```python
from build123d import *

# Parameters (mm, degrees)
SKETCH1_W          = 66.04
SKETCH1_H          = 102.87
EXTRUDE1_DEPTH     = 25.2476
FILLET1_R          = 2.54
SKETCH2_R          = 0.3175
EXTRUDE2_DEPTH     = 5.334
LPATTERN1_COUNT    = 25
LPATTERN1_PITCH    = 2.54
SKETCH3_R          = 0.3175
EXTRUDE3_DEPTH     = 5.334
LPATTERN2_COUNT    = 16
LPATTERN2_PITCH    = 2.54
CUT_EXTRUDE1_START = -5.334
CUT_EXTRUDE1_DEPTH = 5.334
SKETCH5_R          = 2.7051
CUT_EXTRUDE2_DEPTH = 25.654


with BuildPart() as part:
    # Sketch1 → Extrude1 (new body)
    with BuildSketch(Plane(origin=(0, 0, 0), x_dir=(1, 0, 0), z_dir=(0, 1, 0))):
        with Locations((33.02, 51.435)):
            Rectangle(SKETCH1_W, SKETCH1_H)
    extrude(amount=EXTRUDE1_DEPTH)

    # Fillet1
    fillet1_edges = [part.edges().sort_by_distance(p)[0] for p in [
        (0, 12.6238, -102.87),
        (66.04, 12.6238, -102.87),
        (66.04, 12.6238, 0),
        (0, 12.6238, 0),
    ]]
    fillet(fillet1_edges, radius=FILLET1_R)

    # Sketch2 → Extrude2 (add)
    with BuildSketch(Plane.XZ):
        with Locations(Location((56.1848, -20.955, 0), (0, 0, 270))):
            Circle(SKETCH2_R)
        with Locations(Location((58.7248, -20.955, 0), (0, 0, 270))):
            Circle(SKETCH2_R)
    extrude2 = extrude(amount=EXTRUDE2_DEPTH)

    # LPattern1: Extrude2 ×25
    with Locations(*[(0, 0, -i * LPATTERN1_PITCH) for i in range(1, LPATTERN1_COUNT)]):
        add(extrude2)

    # Sketch3 → Extrude3 (add)
    with BuildSketch(Plane.XZ):
        with Locations(Location((8.4328, -69.215, 0), (0, 0, 270))):
            Circle(SKETCH3_R)
        with Locations(Location((10.9728, -69.215, 0), (0, 0, 270))):
            Circle(SKETCH3_R)
    extrude3 = extrude(amount=EXTRUDE3_DEPTH)

    # LPattern2: Extrude3 ×16
    with Locations(*[(0, 0, i * LPATTERN2_PITCH) for i in range(1, LPATTERN2_COUNT)]):
        add(extrude3)

    # Sketch4 → Cut-Extrude1 (cut)
    with BuildSketch(Plane.XZ.offset(CUT_EXTRUDE1_START)):
        with BuildLine():
            Line((53.34, 0), (63.5, 0))
            ThreePointArc((63.5, 0), (65.296051224, -0.743948776), (66.04, -2.54))
            Line((66.04, -2.54), (66.04, -12.7))
            ThreePointArc((66.04, -12.7), (56.838081011, -9.201918989), (53.34, 0))
        make_face()
        with BuildLine():
            Line((12.7, -102.87), (2.54, -102.87))
            ThreePointArc((2.54, -102.87), (0.743948776, -102.126051224), (0, -100.33))
            Line((0, -100.33), (0, -90.17))
            ThreePointArc((0, -90.17), (9.206362116, -93.663637884), (12.7, -102.87))
        make_face()
    extrude(amount=CUT_EXTRUDE1_DEPTH, mode=Mode.SUBTRACT)

    # Sketch5 → Cut-Extrude2 (cut)
    with BuildSketch(Plane.XZ):
        with Locations(Location((33.5788, -5.969, 0), (0, 0, 270))):
            Circle(SKETCH5_R)
        with Locations(Location((33.5788, -94.361, 0), (0, 0, 270))):
            Circle(SKETCH5_R)
    extrude(amount=-CUT_EXTRUDE2_DEPTH, mode=Mode.SUBTRACT)


solid = part.part
```
Check sheet for the modelled part. Datum: model origin and axes. Units: mm. A direction names the side the tool comes from. Coordinates: 2 decimals unless noted, no trailing zeros. Order: outer loops, then holes, each group sorted by start corner. A loop starts at its lowest first (then second) coordinate and runs counter-clockwise, first axis right, second up. Notation, with made-up numbers: M -14.5,-8 L 23.5,-8 A19 ccw 23.5,9 Z; hole C 13,76 d10. An arc over 180 degrees is marked long. One line per question, with ' | ' between items. Start each with the question number.
Item 1: Sectioned sample at B-B on x = 47. Record the cut outline in (y, z).
Item 2: Mould release check, pull along Z, two halves, no side actions. Record for faces 4 (the cylindrical face through (35.41, 12.45, -92.37)), 5 (the flat face through (33, 12, -102.87)), 6 (the cylindrical face through (0.724, 12.801, -0.764)): pulls with the +Z half, pulls with the -Z half, needs draft (parallel to the pull), parting line crosses it, or undercut.
Item 3: Access from +Z, -Z, +X, -X, +Y, -Y to the whole of each face (thin tool, end or side, straight path). Record for faces 1 (the flat face through (33, 12, 0)), 2 (the flat face through (61, 5.334, -5)), 3 (the flat face through (5, 5.334, -98)).
Item 4: Material ranges on line 1 (Z direction, x = 32, y = 6); line 2 (Y direction, x = 62, z = -75.5); line 3 (Z direction, x = 60, y = 2), recorded low to high.
Item 5: Gauge pin test, flat ends, axial feed: P1, Ø4, axis at x = 9, z = -93.5, coming from the -Y side; P2, Ø8.5, axis at x = 33.58, z = -94.36, coming from the +Y side; P3, Ø4, axis at x = 61, z = -9, coming from the -Y side. Record the tip position at first contact, or that the pin passes through.
Item 6: Sectioned sample at A-A on z = -14. Record the cut outline in (x, y), and give its area (3 significant figures).
Answer below:
1) outline: M 0,-102.87 L 25.25,-102.87 L 25.25,0 L 0,0 Z
2) face 4: undercut | face 5: pulls with the -Z half | face 6: pulls with the +Z half
3) face 1: +Z, +X, -X, +Y, -Y | face 2: +Z, +X, -Y | face 3: -Z, -X, -Y
4) line 1: z = -102.87 to -96.56, -92.16 to -8.17, -3.77 to 0 | line 2: y = 0 to 25.25 | line 3: z = -102.87 to -11.47
5) P1: stops at y = 0 | P2: stops at y = 25.25 | P3: stops at y = 5.33
6) outline: M 0,0 L 66.04,0 L 66.04,25.25 L 0,25.25 Z | area: 1,670 mm^2
